Geometry check sheet. Reference: the model listing, model coordinates, mm. A direction names the side the tool comes from. Round coordinates to 2 decimals unless told otherwise and drop trailing zeros. Order: outer loops, then holes, each group sorted by start corner. A loop starts at its lowest first (then second) coordinate and runs counter-clockwise, first axis right, second up.
(1) Go/stop test with flat-tipped pins: pin 1 (10 mm diameter, centred on x = 76, z = 18.5, fed in from -Y); pin 2 (6 mm diameter, centred on y = 18.5, z = 16.5, fed in from +X); pin 3 (12 mm diameter, centred on x = 24.5, y = -46.5, fed in from +Z). Record where each tip stops, or that it passes through.
(2) Material ranges on line 1 along Y through (x, z) = (115.5, 16); line 2 along Z through (x, y) = (167, -40); line 3 along X through (y, z) = (26, 23.25), recorded low to high.
(3) Sectioned sample at C-C (z = 8.25). Record the boundary of the cut face in (x, y).
(4) Set-up check for faces 1 (the face through (50, -37.977, 19)), 2 (the face through (192.374, -6.938, 6.261)): record each of +Z, -Z, +X, -X, +Y, -Y from which the full face is reachable in a straight line by a thin tool's end or side.
from build123d import *

# Parameters (mm, degrees)
F1_DEPTH = 12.7
F2_DEPTH = 12.7


with BuildPart() as f1:
    # F0 (on Top) → F1 (new body)
    with BuildSketch(Plane.XY):
        Polygon((140.862602, 44.572849), (-119.487398, 44.572849), (-119.487398, -37.977151), (223.412602, -37.977151), align=None)
    extrude(amount=F1_DEPTH)

    # F0 (on Top) + F1_face (on face) → F2 (join)
    with BuildSketch(Plane.XY):
        Polygon((140.862602, 44.572849), (-119.487398, 44.572849), (-119.487398, -37.977151), (223.412602, -37.977151), align=None)
        Polygon((223.412602, -37.977151), (-119.487398, -37.977151), (-119.487398, -57.027151), (242.462602, -57.027151), align=None)
    with BuildSketch(Plane(origin=(32.266461, 1.415129, 12.7), x_dir=(1, 0, 0), z_dir=(0, 0, 1))):
        Polygon((108.59614, 43.157719), (-151.75386, 43.157719), (-151.75386, -39.392281), (191.14614, -39.392281), align=None)
    extrude(amount=F2_DEPTH)


solid = f1.part
Answer below:
1. pin 1: stops at y = -37.98
1. pin 2: stops at x = 169.94
1. pin 3: stops at z = 12.7
2. line 1: y = -37.98 to 44.57
2. line 2: z = 0 to 12.7
2. line 3: x = -119.49 to 159.44
3. outline: (-119.49, -57.03) - (242.46, -57.03) - (140.86, 44.57) - (-119.49, 44.57) - close
4. face 1: +Z, +X, -X, -Y
4. face 2: +Z, -Z, +X, +Y
